from build123d import *

# Parameters (mm, degrees)
F1_DEPTH = 50.8
F2_DEPTH = 25.4
F0_R     = 12.7
F3_DEPTH = 31.75


with BuildPart() as f1:
    # F0 (on Front) → F1 (new body)
    with BuildSketch(Plane.XZ):
        with BuildLine():
            Line((-23.4679372151, 35.1908475518), (-38.1188419469, 38.1188242326))
            ThreePointArc((-38.1188419469, 38.1188242326), (-76.2376661794, 0), (-38.1188419469, -38.1188242326))
            Line((-38.1188419469, -38.1188242326), (-23.4679372151, -35.1908475518))
            ThreePointArc((-23.4679372151, -35.1908475518), (-6.4051223354, -21.1491075291), (-1.77143e-05, 0))
            ThreePointArc((-1.77143e-05, 0), (-6.4051223354, 21.1491075291), (-23.4679372151, 35.1908475518))
        make_face()
        with BuildLine():
            ThreePointArc((-55.9794965989, -6.6256709397), (-57.1676480455, -0.2132749771), (-56.123365877, 6.2241158448))
            ThreePointArc((-56.123365877, 6.2241158448), (-38.1188419468, 19.05), (-20.1143180167, 6.2241158448))
            Line((-20.1143180167, 6.2241158448), (-12.8497872502, 6.2241158448))
            Line((-12.8497872502, 6.2241158448), (-12.8497872502, -6.6256709397))
            Line((-12.8497872502, -6.6256709397), (-20.2581872948, -6.6256709397))
            ThreePointArc((-20.2581872948, -6.6256709397), (-38.1188419468, -19.05), (-55.9794965989, -6.6256709397))
        make_face(mode=Mode.SUBTRACT)
    extrude(amount=F1_DEPTH)

    # F0 (on Front) → F2 (join)
    with BuildSketch(Plane.XZ):
        with BuildLine():
            Line((57.2499610198, 19.0594121163), (-23.4679372151, 35.1908475518))
            ThreePointArc((-23.4679372151, 35.1908475518), (-6.4051223354, 21.1491075291), (-1.77143e-05, 0))
            ThreePointArc((-1.77143e-05, 0), (-6.4051223354, -21.1491075291), (-23.4679372151, -35.1908475518))
            Line((-23.4679372151, -35.1908475518), (57.2499610198, -19.0594121163))
            ThreePointArc((57.2499610198, -19.0594121163), (38.1905489035, 0), (57.2499610198, 19.0594121163))
        make_face()
    extrude(amount=F2_DEPTH)

    # F0 (on Front) → F3 (join)
    with BuildSketch(Plane.XZ):
        with BuildLine():
            ThreePointArc((76.309373136, 0), (70.7270005726, 13.4770395529), (57.2499610198, 19.0594121163))
            ThreePointArc((57.2499610198, 19.0594121163), (38.1905489035, 0), (57.2499610198, -19.0594121163))
            ThreePointArc((57.2499610198, -19.0594121163), (70.7270005726, -13.4770395529), (76.309373136, 0))
        make_face()
        with Locations((57.2499610198, 0)):
            Circle(F0_R, mode=Mode.SUBTRACT)
    extrude(amount=F3_DEPTH)


solid = f1.part
Geometry check sheet. Reference: the model listing, model coordinates, mm. A direction names the side the tool comes from. Give positions to 0.01 mm unless a question says otherwise; leave off trailing zeros. Write each loop counter-clockwise with the first axis right and the second up, starting at its lowest first coordinate (ties: lowest second). Pieces come first, ordered by that corner, then holes. Notation, with made-up numbers: M 11,29 L 24,29 A16 cw 24,45 Z; hole C 55,14.25 d8. An arc over 180 degrees is marked long. Answer as CSV lines item,"result". Start each with the question number.
Q1. Section check D-D, the plane y = -37. Record the cut outline in (x, z), then the cut area to 3 significant figures.
Q2. Material ranges on L1, parallel to X at y = -3, z = -16; L2, parallel to X at y = -14.5, z = -17.5; L3, parallel to Y at x = -7, z = 28.5, recorded low to high.
Q3. Go/stop test with flat-tipped pins: pin 1 (1 mm diameter, centred on y = -31.5, z = 20, fed in from +X); pin 2 (4 mm diameter, centred on x = -16, y = -8.5, fed in from -Z); pin 3 (3 mm diameter, centred on x = -42, y = -25, fed in from -Z). Record where each tip stops, or that it passes through.
Q4. Section check A-A, the plane y = -27.5. Record the cut outline in (x, z).
Q5. Tool access check on faces 4 (the face through (70, -31.75, -4)), 5 (the face through (-17, -25, -6.626)), 6 (the face through (-56, -50.8, -8)). Record the directions out of +Z, -Z, +X, -X, +Y, -Y that give a thin tool (end or side, any length) a straight path to the whole face; none if there is none.
Q6. Release check for a two-part mould opening along X. For faces 1 (the face through (-76.23, -25.04, 0.84)), 2 (the face through (-1, 0, 1)), 3 (the face through (-17, -25, 6.224)) record: pulls with the +X half, pulls with the -X half, needs draft (parallel to the pull), parting line crosses it, or undercut.
Q7. Section check C-C, the plane x = 53.5. Record the cut outline in (y, z).
Q8. Section check B-B, the plane y = -4. Record the cut outline in (x, z), then the cut area to 3 significant figures.
Geometry says:
1,outline,"M -38.12,-38.12 L -23.47,-35.19 A38.12 ccw -23.47,35.19 L -38.12,38.12 A38.12 ccw Z; hole M -20.26,-6.63 L -12.85,-6.63 L -12.85,6.22 L -20.11,6.22 A19.05 ccw long Z"
1,area,"3,330 mm^2"
2,L1,"-72.72 to -48.46, -27.78 to 67.61"
2,L2,"-71.98 to -45.65, -30.59 to 64.8"
2,L3,"-25.4 to 0"
3,pin 1,"x = -5.37"
3,pin 2,"z = -34.1"
3,pin 3,"z = -38.04"
4,outline,"M -38.12,-38.12 L -23.47,-35.19 A38.12 ccw -23.47,35.19 L -38.12,38.12 A38.12 ccw Z; C 57.25,0 d38.12; hole M -20.26,-6.63 L -12.85,-6.63 L -12.85,6.22 L -20.11,6.22 A19.05 ccw long Z; hole C 57.25,0 d25.4"
5,face 4,"+Z, -Z, +X, -Y"
5,face 5,"+Y, -Y"
5,face 6,"+Z, -Z, +X, -X, -Y"
6,face 1,"pulls with the -X half"
6,face 2,"needs draft"
6,face 3,"undercut"
7,outline,"M -31.75,-18.69 L -25.4,-18.69 L -25.4,-19.81 L 0,-19.81 L 0,-12.13 L -31.75,-12.13 Z; M -31.75,12.13 L 0,12.13 L 0,19.81 L -25.4,19.81 L -25.4,18.69 L -31.75,18.69 Z"
8,outline,"M -38.12,-38.12 L 57.25,-19.06 A19.06 ccw 57.25,19.06 L -38.12,38.12 A38.12 ccw Z; hole M -20.26,-6.63 L -12.85,-6.63 L -12.85,6.22 L -20.11,6.22 A19.05 ccw long Z; hole C 57.25,0 d25.4"
8,area,"6,570 mm^2"
